CAD build for the part. Positions are in the model's coordinates, mm. A direction names the side the tool comes from. Coordinates: 2 decimals unless noted, no trailing zeros. Loops run counter-clockwise (first coordinate to the right, second up) from the corner with the lowest first, then second, coordinate; pieces in that order, holes last. Notation, with made-up numbers: (61, -11) -> (98, -11) arc R28 cw to (98, 7) -> close; hole circle Ø11 at (-23, -35.5). An arc over 180 degrees is marked (long way). Write each question's results on one line, items separated by ' | '.
from build123d import *

# Parameters (mm, degrees)
IZIM1_W                     = 6
IZIM1_H                     = 6
Y_KSEKLIK_EKSTR_ZYON1_DEPTH = 3.3
IZIM2_W                     = 6
IZIM2_H                     = 6
Y_KSEKLIK_EKSTR_ZYON2_DEPTH = 0.1
IZIM3_W                     = 3
IZIM3_H                     = 0.2
KES_EKSTR_ZYON1_DEPTH       = 1.5
IZIM4_W                     = 2
IZIM4_H                     = 0.2
KES_EKSTR_ZYON2_DEPTH       = 8.475961477
IZIM5_R                     = 1.7
Y_KSEKLIK_EKSTR_ZYON3_DEPTH = 3.4
DRAFT4_ANGLE                = 1
IZIM6_R                     = 0.6
Y_KSEKLIK_EKSTR_ZYON4_DEPTH = 0.5
Y_KSEKLIK_EKSTR_ZYON5_DEPTH = 0.35
L_O_ALTMA1_COUNT            = 2
L_O_ALTMA1_PITCH            = 4.5


with BuildPart() as part:
    # Çizim1 → Yükseklik-Ekstrüzyon1 (new body)
    with BuildSketch(Plane(origin=(0, 0, 0), x_dir=(1, 0, 0), z_dir=(0, 1, 0))):
        Rectangle(IZIM1_W, IZIM1_H)
    extrude(amount=-Y_KSEKLIK_EKSTR_ZYON1_DEPTH)

    # Çizim2 → Yükseklik-Ekstrüzyon2 (add)
    with BuildSketch(Plane(origin=(0, 0, 0), x_dir=(1, 0, 0), z_dir=(0, 1, 0))):
        Rectangle(IZIM2_W, IZIM2_H)
    extrude(amount=Y_KSEKLIK_EKSTR_ZYON2_DEPTH)

    # Çizim3 → Kes-Ekstrüzyon1 (cut)
    with BuildSketch(Plane.XY.offset(3)):
        with Locations((0, -3.2)):
            Rectangle(IZIM3_W, IZIM3_H)
    kes_ekstr_zyon1 = extrude(amount=-KES_EKSTR_ZYON1_DEPTH, mode=Mode.SUBTRACT)

    # Aynalama1: Kes-Ekstrüzyon1 across plane
    add(kes_ekstr_zyon1.mirror(Plane.XY), mode=Mode.SUBTRACT)

    # Çizim4 → Kes-Ekstrüzyon2 (cut, through all)
    with BuildSketch(Plane.ZY.offset(3)):
        with Locations((0, -3.2)):
            Rectangle(IZIM4_W, IZIM4_H)
    extrude(amount=-KES_EKSTR_ZYON2_DEPTH, mode=Mode.SUBTRACT)

    # Çizim5 → Yükseklik-Ekstrüzyon3 (add)
    with BuildSketch(Plane(origin=(0, 0.1, 0), x_dir=(1, 0, 0), z_dir=(0, 1, 0))):
        with Locations(Location((0, 0, 0), (0, 0, 270))):
            Circle(IZIM5_R)
    extrude(amount=Y_KSEKLIK_EKSTR_ZYON3_DEPTH)

    # Draft4
    draft4_faces = [part.faces().sort_by_distance(p)[0] for p in [
        (0, 1.8, -1.7),
    ]]
    draft(draft4_faces, Plane.ZX.offset(3.5), DRAFT4_ANGLE)

    # Çizim6 → Yükseklik-Ekstrüzyon4 (add)
    with BuildSketch(Plane(origin=(0, 0.1, 0), x_dir=(1, 0, 0), z_dir=(0, 1, 0))):
        with Locations(Location((-2.3, 2.3, 0), (0, 0, 270))):
            Circle(IZIM6_R)
        with Locations(Location((2.3, 2.3, 0), (0, 0, 90))):
            Circle(IZIM6_R)
        with Locations(Location((2.3, -2.3, 0), (0, 0, 270))):
            Circle(IZIM6_R)
        with Locations(Location((-2.3, -2.3, 0), (0, 0, 90))):
            Circle(IZIM6_R)
    extrude(amount=Y_KSEKLIK_EKSTR_ZYON4_DEPTH)

    # Çizim8 → Yükseklik-Ekstrüzyon5 (add, symmetric)
    with BuildSketch(Plane.XY.offset(2.25)):
        Polygon((-3, -2.63511714), (-3.756588195, -2.63511714), (-3.70725074, -3.782570711), (-4.005822093, -5.10919798), (-3.4, -6.825693909), (-3.4, -8.597874756), (-3.1, -8.597874756), (-3.1, -6.774306091), (-3.694177907, -5.09080202), (-3.405814351, -3.809530548), (-3.443411805, -2.93511714), (-3, -2.93511714), align=None)
        Polygon((3, -2.93511714), (3.443411805, -2.93511714), (3.405814351, -3.809530548), (3.694177907, -5.09080202), (3.1, -6.774306091), (3.1, -8.597874756), (3.4, -8.597874756), (3.4, -6.825693909), (4.005822093, -5.10919798), (3.70725074, -3.782570711), (3.756588195, -2.63511714), (3, -2.63511714), align=None)
    y_kseklik_ekstr_zyon5 = extrude(amount=Y_KSEKLIK_EKSTR_ZYON5_DEPTH, both=True)

    # LÇoğaltma1: Yükseklik-Ekstrüzyon5 ×2
    with Locations(*[(0, 0, -i * L_O_ALTMA1_PITCH) for i in range(1, L_O_ALTMA1_COUNT)]):
        add(y_kseklik_ekstr_zyon5)


solid = part.part
1) Drill centre lines: L1, parallel to Y at x = -2.75, z = -1.8; L2, parallel to Y at x = 2.75, z = 0.3; L3, parallel to X at y = -2.5, z = 0.05. Where is each one in solid material? Low to high. Write a range as from..to.
Outcome:
L1: y = -3.3..0.1 | L2: y = -3.1..0.1 | L3: x = -3..3
2) Slice it at D-D (y = 0.75). Write the cut outline in (x, z).
Outcome:
outline: circle Ø3.5 at (0, 0)
3) Slice it at B-B (y = -0.5). Write the cut outline in (x, z), then the cut area to 3 significant figures.
Outcome:
outline: (-3, -3) -> (3, -3) -> (3, 3) -> (-3, 3) -> close | area: 36.0 mm^2
4) Pin check, flat tips, straight feed: pin 1 (1.3 mm diameter, centred on x = -2, z = 2, fed in from +Y); pin 2 (1.6 mm diameter, centred on x = 1, z = 2.5, fed in from -Y); pin 3 (2.5 mm diameter, centred on y = -1.5, z = 0, fed in from -X); pin 4 (3 mm diameter, centred on x = -0.5, y = -7, fed in from +Z). Stop position of each tip, or through.
Outcome:
pin 1: stops at y = 0.6 | pin 2: stops at y = -3.3 | pin 3: stops at x = -3 | pin 4: passes through
5) Slice it at A-A (x = 2.3). Write the cut outline in (y, z), then the cut area to 3 significant figures.
Outcome:
outline: (-3.3, -3) -> (0.1, -3) -> (0.1, -2.9) -> (0.6, -2.9) -> (0.6, -1.7) -> (0.1, -1.7) -> (0.1, 1.7) -> (0.6, 1.7) -> (0.6, 2.9) -> (0.1, 2.9) -> (0.1, 3) -> (-3.3, 3) -> (-3.3, 1) -> (-3.1, 1) -> (-3.1, -1) -> (-3.3, -1) -> close | area: 21.2 mm^2
6) Two-plate mould, pull along Z, no slides. Class faces 4 (the flat face through (0, -2, 3)), 5 (the flat face through (-2, 0.6, -2)), 6 (the cylindrical face through (1.77, 0.35, 2.58)): pulls with the +Z half, pulls with the -Z half, needs draft (parallel to the pull), parting line crosses it, or undercut.
Outcome:
face 4: pulls with the +Z half | face 5: needs draft | face 6: undercut
7) Which spindle directions (+Z, -Z, +X, -X, +Y, -Y) get a long thin tool onto all of the face, cutting with end or side? Do faces 1 (the flat face through (0, -3.1, 2)), 2 (the cylindrical face through (-1.714, 0.347, 2.43)), 3 (the flat face through (0, -3.3, -1.3)). Say none if no direction does.
Outcome:
face 1: +Z, -Y | face 2: +Y | face 3: +Z, -Z, -Y
8) Slice it at C-C (x = -2). Write the cut outline in (y, z), then the cut area to 3 significant figures.
Outcome:
outline: (-3.3, -3) -> (0.1, -3) -> (0.1, -2.82) -> (0.6, -2.82) -> (0.6, -1.78) -> (0.1, -1.78) -> (0.1, 1.78) -> (0.6, 1.78) -> (0.6, 2.82) -> (0.1, 2.82) -> (0.1, 3) -> (-3.3, 3) -> (-3.3, 1) -> (-3.1, 1) -> (-3.1, -1) -> (-3.3, -1) -> close | area: 21.0 mm^2
